Answer from the drawing. Dimensions are ordinates in mm from the lowest x, y and z of the part. Coordinates: 2 decimals unless noted, no trailing zeros. Write each loop counter-clockwise with the first axis right and the second up, starting at its lowest first coordinate (ties: lowest second). Pieces come first, ordered by that corner, then holes.
1) The part is cut by section B-B (x = 10). Determine the outline of the cut face in (y, z), then the cut area to 3 significant figures.
2) The part is cut by section A-A (y = 125). Determine the outline of the cut face in (x, z), then the cut area to 3 significant figures.
3) Each of these flat-tipped pins is pushed along its axis until it touches: pin 1 Ø5 at (y, z) = (90.5, 8.5) entering from -X; pin 2 Ø5.5 at (x, y) = (10, 240) entering from +Z. Where does it stop, or does it pass through?
4) Find the intervals of material crossed by line 1 (Y direction, x = 10, z = 2.5); line 2 (X direction, y = 240, z = 7.5); line 3 (Y direction, x = 7.75, z = 9.25), in increasing order.
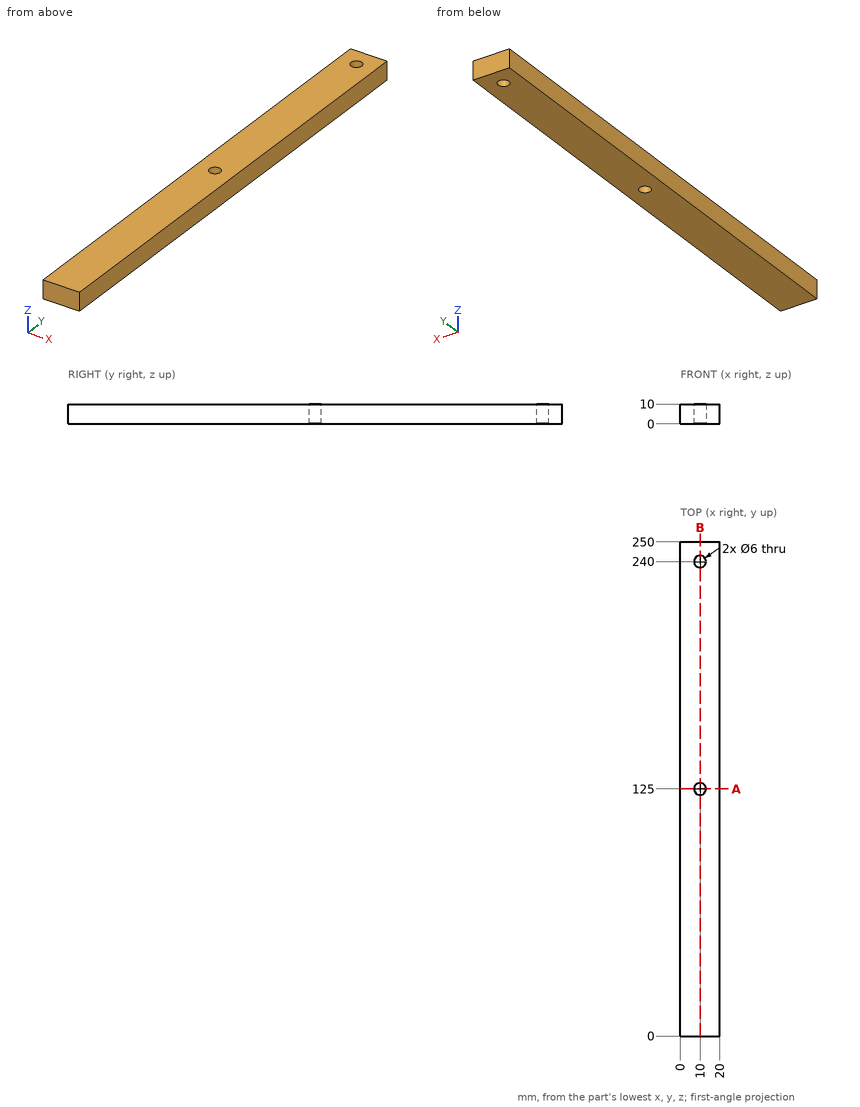
Reported:
1. outline: (0, 0) - (122, 0) - (122, 10) - (0, 10) - close; (128, 0) - (237, 0) - (237, 10) - (128, 10) - close; (243, 0) - (250, 0) - (250, 10) - (243, 10) - close
1. area: 2,380 mm2
2. outline: (0, 0) - (7, 0) - (7, 10) - (0, 10) - close; (13, 0) - (20, 0) - (20, 10) - (13, 10) - close
2. area: 140 mm2
3. pin 1: stops at x = 0
3. pin 2: passes through
4. line 1: y = 0 to 122, 128 to 237, 243 to 250
4. line 2: x = 0 to 7, 13 to 20
4. line 3: y = 0 to 123.02, 126.98 to 238.02, 241.98 to 250
